Part model, mm, in its own coordinate system. Round coordinates to 2 decimals unless told otherwise and drop trailing zeros.
```python
from build123d import *

# Parameters (mm, degrees)
F0_W     = 240
F0_H     = 30
F0_R     = 2
F1_DEPTH = 4


with BuildPart() as f1:
    # F0 (on Front) → F1 (new body)
    with BuildSketch(Plane.XZ):
        Rectangle(F0_W, F0_H)
        with Locations((-110, 0)):
            Circle(F0_R, mode=Mode.SUBTRACT)
        with BuildLine():
            ThreePointArc((105, 0), (103.5355339059, -3.5355339059), (100, -5))
            Line((100, -5), (80, -5))
            Line((80, -5), (60, -5))
            Line((60, -5), (40, -5))
            Line((40, -5), (20.0000000117, -5))
            Line((20.0000000117, -5), (-1.87e-08, -5))
            Line((-1.87e-08, -5), (-19.9999999883, -5))
            Line((-19.9999999883, -5), (-40, -5))
            Line((-40, -5), (-60, -5))
            Line((-60, -5), (-80, -5))
            Line((-80, -5), (-100, -5))
            ThreePointArc((-100, -5), (-105, 0), (-100, 5))
            Line((-100, 5), (-80, 5))
            Line((-80, 5), (-60, 5))
            Line((-60, 5), (-40, 5))
            Line((-40, 5), (-20, 5))
            Line((-20, 5), (-1.17e-08, 5))
            Line((-1.17e-08, 5), (20, 5))
            Line((20, 5), (40, 5))
            Line((40, 5), (60, 5))
            Line((60, 5), (80, 5))
            Line((80, 5), (100, 5))
            ThreePointArc((100, 5), (103.5355339059, 3.5355339059), (105, 0))
        make_face(mode=Mode.SUBTRACT)
        with Locations((110, 0)):
            Circle(F0_R, mode=Mode.SUBTRACT)
        with BuildLine():
            Line((-100, -5), (-80, -5))
            ThreePointArc((-80, -5), (-85, 0), (-80, 5))
            Line((-80, 5), (-100, 5))
            ThreePointArc((-100, 5), (-96.4644660941, 3.5355339059), (-95, 0))
            ThreePointArc((-95, 0), (-96.4644660941, -3.5355339059), (-100, -5))
        make_face()
        with BuildLine():
            Line((-80, -5), (-60, -5))
            ThreePointArc((-60, -5), (-65, 0), (-60, 5))
            Line((-60, 5), (-80, 5))
            ThreePointArc((-80, 5), (-76.4644660941, 3.5355339059), (-75, 0))
            ThreePointArc((-75, 0), (-76.4644660941, -3.5355339059), (-80, -5))
        make_face()
        with BuildLine():
            Line((-60, -5), (-40, -5))
            ThreePointArc((-40, -5), (-45, 0), (-40, 5))
            Line((-40, 5), (-60, 5))
            ThreePointArc((-60, 5), (-56.4644660941, 3.5355339059), (-55, 0))
            ThreePointArc((-55, 0), (-56.4644660941, -3.5355339059), (-60, -5))
        make_face()
        with BuildLine():
            Line((-40, -5), (-19.9999999883, -5))
            ThreePointArc((-19.9999999883, -5), (-25, -5.8e-09), (-20, 5))
            Line((-20, 5), (-40, 5))
            ThreePointArc((-40, 5), (-36.4644660941, 3.5355339059), (-35, 0))
            ThreePointArc((-35, 0), (-36.4644660941, -3.5355339059), (-40, -5))
        make_face()
        with BuildLine():
            Line((-19.9999999883, -5), (-1.87e-08, -5))
            ThreePointArc((-1.87e-08, -5), (-5, 3.5e-09), (-1.17e-08, 5))
            Line((-1.17e-08, 5), (-20, 5))
            ThreePointArc((-20, 5), (-16.4644660941, 3.5355339059), (-15, 0))
            ThreePointArc((-15, 0), (-16.4644660899, -3.5355339018), (-19.9999999883, -5))
        make_face()
        with BuildLine():
            Line((-1.87e-08, -5), (20.0000000117, -5))
            ThreePointArc((20.0000000117, -5), (15, -5.8e-09), (20, 5))
            Line((20, 5), (-1.17e-08, 5))
            ThreePointArc((-1.17e-08, 5), (3.5355339018, 3.5355339101), (5, 0))
            ThreePointArc((5, 0), (3.5355338993, -3.5355339125), (-1.87e-08, -5))
        make_face()
        with BuildLine():
            Line((20.0000000117, -5), (40, -5))
            ThreePointArc((40, -5), (35, 0), (40, 5))
            Line((40, 5), (20, 5))
            ThreePointArc((20, 5), (23.5355339059, 3.5355339059), (25, 0))
            ThreePointArc((25, 0), (23.5355339101, -3.5355339018), (20.0000000117, -5))
        make_face()
        with BuildLine():
            Line((40, -5), (60, -5))
            ThreePointArc((60, -5), (55, 0), (60, 5))
            Line((60, 5), (40, 5))
            ThreePointArc((40, 5), (43.5355339059, 3.5355339059), (45, 0))
            ThreePointArc((45, 0), (43.5355339059, -3.5355339059), (40, -5))
        make_face()
        with BuildLine():
            Line((60, -5), (80, -5))
            ThreePointArc((80, -5), (75, 0), (80, 5))
            Line((80, 5), (60, 5))
            ThreePointArc((60, 5), (63.5355339059, 3.5355339059), (65, 0))
            ThreePointArc((65, 0), (63.5355339059, -3.5355339059), (60, -5))
        make_face()
        with BuildLine():
            Line((80, -5), (100, -5))
            ThreePointArc((100, -5), (95, 0), (100, 5))
            Line((100, 5), (80, 5))
            ThreePointArc((80, 5), (83.5355339059, 3.5355339059), (85, 0))
            ThreePointArc((85, 0), (83.5355339059, -3.5355339059), (80, -5))
        make_face()
    extrude(amount=F1_DEPTH)


solid = f1.part
```
Q1. Cut at A-A on y = -2. State how many separate pieces and enclosed holes the cut face has, plus the area to 3 significant figures.
Values follow:
separate pieces: 1
enclosed holes: 13
area: 6,310 mm2
Q2. Mould opens along Z. For faces 1 (the flat face through (-2, -2, 15)), 2 (the flat face through (-120, -2, 0)), 3 (the cylindrical face through (108, -2, 0)) say: +Z half, -Z half, draft (parallel to the pull), parting line (faces both ways), or undercut.
Values follow:
face 1: +Z half
face 2: draft
face 3: undercut
Q3. Wall check: L1, parallel to Z at x = -110, y = -3.05; L2, parallel to Z at x = -41, y = -2.3. Give the ranges that are in metal, low to high.
Values follow:
L1: z = -15 to -2, 2 to 15
L2: z = -15 to -4.9, 4.9 to 15
